from build123d import *

# Parameters (mm, degrees)
SKETCH_1_W          = 10
SKETCH_1_H          = 20
EXTRUDE_1_DEPTH     = 1251
SKETCH_2_W          = 8
SKETCH_2_H          = 19
CUT_EXTRUDE_1_DEPTH = 2503


with BuildPart() as part:
    # 草图1 → 凸台-拉伸1 (new body)
    with BuildSketch(Plane.XY):
        Rectangle(SKETCH_1_W, SKETCH_1_H)
    extrude(amount=EXTRUDE_1_DEPTH)

    # 草图2 → 切除-拉伸1 (cut)
    with BuildSketch(Plane(origin=(0, 0, 0), x_dir=(-1, 0, 0), z_dir=(0, 0, -1))):
        with Locations((0, 10)):
            Rectangle(SKETCH_2_W, SKETCH_2_H)
        with Locations((0, -10)):
            Rectangle(SKETCH_2_W, SKETCH_2_H)
    extrude(amount=-CUT_EXTRUDE_1_DEPTH, mode=Mode.SUBTRACT)


solid = part.part
Could you check a few things on this model? Use its own coordinates, in mm. Coordinates: 2 decimals unless noted, no trailing zeros. Write each loop counter-clockwise with the first axis right and the second up, starting at its lowest first coordinate (ties: lowest second). Pieces come first, ordered by that corner, then holes. Notation, with made-up numbers: (-7.5, 33.25) - (16.5, 33.25) arc R18 cw to (16.5, 37.25) - close; hole circle Ø9 at (-24.5, -20.75). An arc over 180 degrees is marked (long way). Put each result on its own line as item: value. Start each with the question number.
Q1. I want a section at A-A on y = 6. Write out the boundary of the cut face in (x, z), plus the area to 3 significant figures.
Q2. I want a section at B-B on z = 139. Write out the boundary of the cut face in (x, y).
Q3. Please list where these lines run through material, in increasing order: L1, parallel to X at y = 2, z = 637; L2, parallel to Y at x = 3.5, z = 886.
Q4. I want a section at C-C on x = -0.5. Write out the boundary of the cut face in (y, z).
Q5. I'm going to push flat-ended pins straight in: P1, Ø1.5, axis at x = 2.5, z = 689, coming from the -Y side; P2, Ø5, axis at x = 0, z = 146, coming from the +Y side. Where does each tip first touch, or does it pass through?
Checks:
1. outline: (-5, 0) - (-4, 0) - (-4, 1251) - (-5, 1251) - close; (4, 0) - (5, 0) - (5, 1251) - (4, 1251) - close
1. area: 2,500 mm²
2. outline: (-5, -10) - (-4, -10) - (-4, -0.5) - (4, -0.5) - (4, -10) - (5, -10) - (5, 10) - (4, 10) - (4, 0.5) - (-4, 0.5) - (-4, 10) - (-5, 10) - close
3. L1: -5 to -4, 4 to 5
3. L2: -0.5 to 0.5
4. outline: (-0.5, 0) - (0.5, 0) - (0.5, 1251) - (-0.5, 1251) - close
5. P1: y = -0.5
5. P2: y = 0.5
